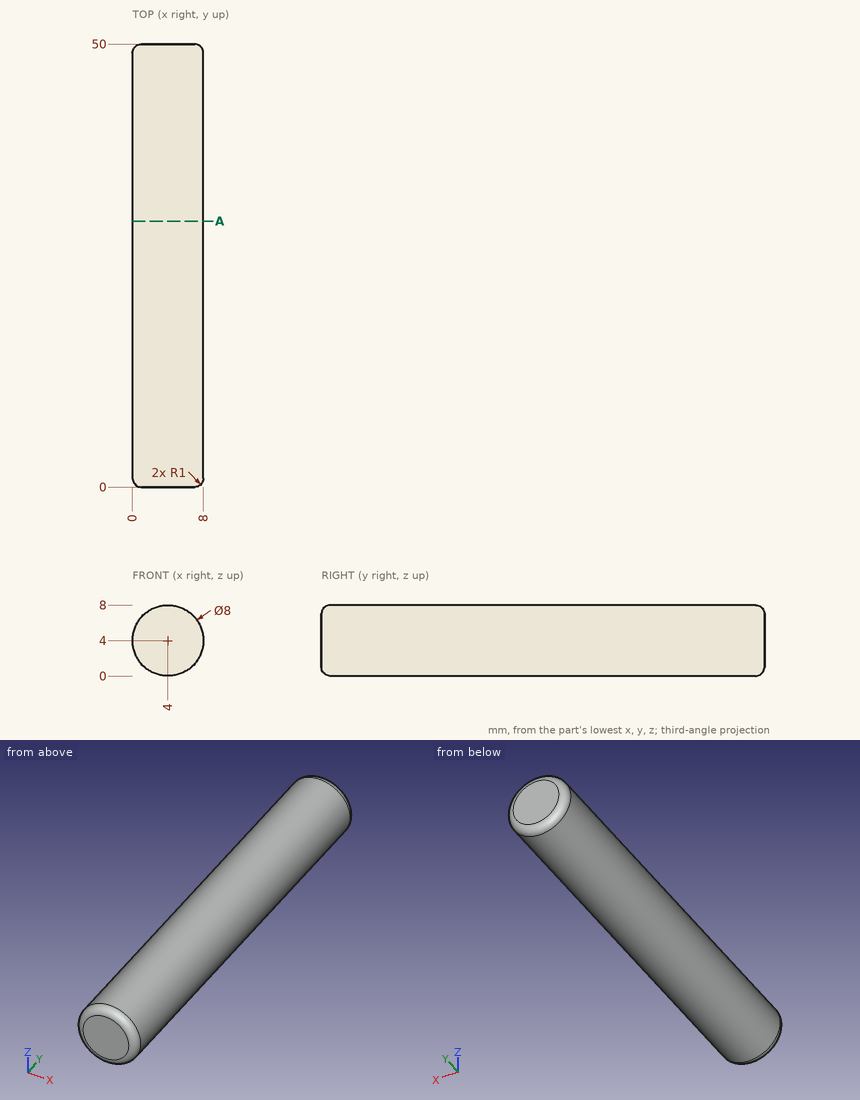
Verification items for this drawing (mm, ordinates from the low corner). Coordinates: 2 decimals unless noted, no trailing zeros. Loops run counter-clockwise (first coordinate to the right, second up) from the corner with the lowest first, then second, coordinate; pieces in that order, holes last. Notation, with made-up numbers: (-15.5, 51.25) -> (23.5, 51.25) arc R19 cw to (23.5, 59.25) -> close; hole circle Ø5 at (85.5, 18). An arc over 180 degrees is marked (long way). Answer in a Markdown table with one row per item. Add a question column.
1. Material ranges on probe 1 along X at (y, z) = (4.5, 4.25); probe 2 along Y at (x, z) = (1.25, 6.25); probe 3 along X at (y, z) = (20.5, 5), recorded low to high. Write a range as [from, to].
2. Section check A-A, the plane y = 30. Enter the section's corners in (x, z).
3. Depth check by flat-ended pin: P1, Ø4, axis at y = 14, z = 7, coming from the +X side. Enter the tip coordinate at first touch or a pass-through.
Derived:
| question | item | result |
|---|---|---|
| 1 | probe 1 | x = [0.01, 7.99] |
| 1 | probe 2 | y = [0.17, 49.83] |
| 1 | probe 3 | x = [0.13, 7.87] |
| 2 | outline | circle Ø8 at (4, 4) |
| 3 | P1 | stops at x = 7.87 |
